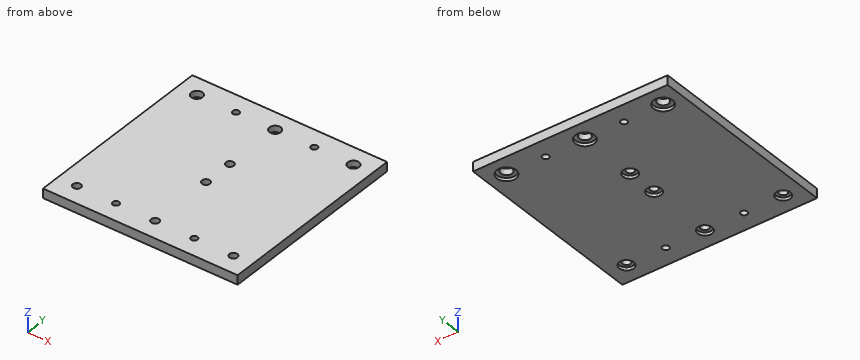
Autodesk Inventor part; units mm, degrees
ref_plane "YZ Plane" through (0, 0, 0) normal (1, 0, 0) x (0, 1, 0)
ref_plane "XZ Plane" through (0, 0, 0) normal (0, 1, 0) x (-1, 0, 0)
ref_plane "XY Plane" through (0, 0, 0) normal (0, 0, 1) x (1, 0, 0)
sketch "Sketch1" plane through (0, 0, 0) normal (0, 0, 1) x (1, 0, 0)
  line L0 (97.2346, 27.952) -> (-27.7654, 27.952)
  line L1 (-27.7654, 27.952) -> (-27.7654, -97.248)
  line L2 (-27.7654, -97.248) -> (97.2346, -97.248)
  line L3 (97.2346, -97.248) -> (97.2346, 27.952)
  line L4 (85.1346, 27.952) -> (85.1346, -97.248) construction
  line L5 (-15.4654, 27.952) -> (-15.4654, -97.248) construction
  line L6 (-37.3152, 15.652) -> (117.1466, 15.652) construction
  line L7 (115.2487, -84.948) -> (-56.3615, -84.948) construction
  line L8 (34.8346, -156.7023) -> (34.8346, 57.8793) construction
  line L9 (59.9846, 68.2484) -> (59.9846, -132.2245) construction
  line L10 (9.6846, 55.4717) -> (9.6846, -128.574) construction
  point P0 (0, 0)
  point P1 (-65.7997, 171.2688)
  point P2 (85.1346, -84.948)
  point P3 (85.1346, 15.652)
  point P4 (-15.4654, 15.652)
  point P5 (-15.4654, -84.948)
  point P6 (34.8346, -84.948)
  point P7 (34.8346, 15.652)
  point P8 (59.9846, 15.652)
  point P9 (9.6846, 15.652)
  point P10 (59.9846, -84.948)
  point P11 (9.6846, -84.948)
  dimension "d0" = 125
  dimension "d1" = 125.2
  dimension "d6" = 100.6
  dimension "d48" = 12.3
  dimension "d49" = 100.6
  dimension "d50" = 50.3
  dimension "d72" = 25.15
  dimension "d73" = 25.15
extrude "Extrusion1" add sketch "Sketch1" along normal blind 6
hole "Hole6" at (85.1346, -84.948, 0) at (34.8346, -84.948, 0) at (-15.4654, -84.948, 0) direction (0, 0, 1) diameter 5.1 end through all counterbore diameter 9.2 counterbore depth 2
sketch "Sketch2" plane through (0, 0, 6) normal (0, 0, 1) x (1, 0, 0)
  line L0 (86.1945, -57.9789) -> (32.1694, -57.9789) construction
  line L1 (32.1694, -57.9789) -> (32.1694, -50.1092) construction
  line L2 (32.1694, -50.1092) -> (86.1945, -50.1092) construction
  line L3 (86.1945, -50.1092) -> (86.1945, -57.9789) construction
  point P0 (0, 0)
sketch "Sketch3" plane through (0, 0, 0) normal (0, 0, -1) x (-1, 0, 0)
  point P0 (0, 0)
hole "Hole7" at (85.1346, 15.652, 0) at (34.8346, 15.652, 0) at (-15.4654, 15.652, 0) direction (0, 0, 1) diameter 7.2 end through all counterbore diameter 12.25 counterbore depth 2
sketch "Sketch5" plane through (0, 0, 0) normal (0, 0, -1) x (-1, 0, 0)
  point P0 (0, 0)
  point P1 (-34.7346, -22.248)
  point P2 (-34.7346, -42.248)
hole "Hole8" at (34.7346, -22.248, 0) at (34.7346, -42.248, 0) direction (0, 0, 1) diameter 5.1 end through all counterbore diameter 9.2 counterbore depth 2
hole "Hole9" at (59.9846, 15.652, 0) at (9.6846, 15.652, 0) at (59.9846, -84.948, 0) at (9.6846, -84.948, 0) direction (0, 0, 1) diameter 4.2 end through all
equation "\"d72\" = 0.5 * d50"
equation "\"d73\" = 0.5 * d50"
properties part number "X axis carriage small_3DPrint"
Could you check a few things on this model? Use its own coordinates, in mm. Give positions to 0.01 mm unless a question says otherwise; leave off trailing zeros. Order: outer loops, then holes, each group sorted by start corner. A loop starts at its lowest first (then second) coordinate and runs counter-clockwise, first axis right, second up.
1. Suppose I cut it at A-A (y = -41.5). Write out the boundary of the cut face in (x, z).
Answers below:
outline: (-27.77, 0) - (30.2, 0) - (30.2, 2) - (32.3, 2) - (32.3, 6) - (-27.77, 6) - close; (37.17, 2) - (39.27, 2) - (39.27, 0) - (97.23, 0) - (97.23, 6) - (37.17, 6) - close
2. I need wall thicknesses on L1, parallel to X at y = 16, z = 4.3; L2, parallel to X at y = -42, z = 4.25; L3, parallel to Y at x = -16.5, z = 4.85. Which ranges of each line are inside material? Lowest first, please.
Answers below:
L1: x = -27.77 to -19.05, -11.88 to 7.61, 11.76 to 31.25, 38.42 to 57.91, 62.06 to 81.55, 88.72 to 97.23
L2: x = -27.77 to 32.2, 37.27 to 97.23
L3: y = -97.25 to -87.28, -82.62 to 12.2, 19.1 to 27.95
3. For pin 1 (4.5 mm diameter, centred on x = 36, y = -86, fed in from -Z); pin 2 (4 mm diameter, centred on x = 59.98, y = -84.95, fed in from +Z), each with a flat end and sliding along its axis, tell me the tip position at first contact or that it passes through.
Answers below:
pin 1: stops at z = 2
pin 2: passes through
4. Suppose I cut it at B-B (z = 3.8). State how many separate pieces and enclosed holes the cut face has, plus the area to 3 significant figures.
Answers below:
separate pieces: 1
enclosed holes: 12
area: 15,400 mm2
